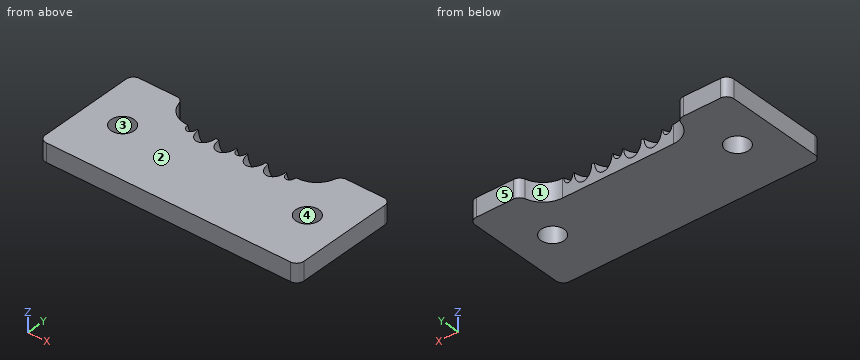
```python
from build123d import *

# Parameters (mm, degrees)
SKETCH1_R               = 3.96875
BOSS_EXTRUDE1_DEPTH     = 6.35
SKETCH2_R               = 3
SKETCH2_R_2             = 1.5875
CUT_EXTRUDE1_DEPTH      = 22.326340521
CUT_EXTRUDE1_DEPTH_BACK = 11.104555903


with BuildPart() as part:
    # Sketch1 → Boss-Extrude1 (new body)
    with BuildSketch(Plane.XY):
        with BuildLine():
            ThreePointArc((17.691011583, 36.198659004), (20.503728332, 31.849390129), (25.4, 30.16))
            Line((25.4, 30.16), (63.5, 30.16))
            ThreePointArc((63.5, 30.16), (68.396271668, 31.849390129), (71.208988417, 36.198659004))
            ThreePointArc((71.208988417, 36.198659004), (72.094604522, 37.568076156), (73.636251773, 38.1))
            Line((73.636251773, 38.1), (86.4, 38.1))
            ThreePointArc((86.4, 38.1), (88.167766953, 37.367766953), (88.9, 35.6))
            Line((88.9, 35.6), (88.9, 2.5))
            ThreePointArc((88.9, 2.5), (88.167766953, 0.732233047), (86.4, 0))
            Line((86.4, 0), (2.5, 0))
            ThreePointArc((2.5, 0), (0.732233047, 0.732233047), (0, 2.5))
            Line((0, 2.5), (0, 35.6))
            ThreePointArc((0, 35.6), (0.732233047, 37.367766953), (2.5, 38.1))
            Line((2.5, 38.1), (15.263748227, 38.1))
            ThreePointArc((15.263748227, 38.1), (16.805395478, 37.568076156), (17.691011583, 36.198659004))
        make_face()
        with Locations((12.7, 19.05)):
            Circle(SKETCH1_R, mode=Mode.SUBTRACT)
        with Locations((76.2, 19.05)):
            Circle(SKETCH1_R, mode=Mode.SUBTRACT)
    extrude(amount=BOSS_EXTRUDE1_DEPTH)

    # Sketch2 → Cut-Extrude1 (cut, two sides)
    with BuildSketch(Plane(origin=(0, 11.905, -11.905), x_dir=(1, 0, 0), z_dir=(0, -0.707106781, 0.707106781))) as cut_extrude1_sk:
        with Locations((49.45, 25.816468581)):
            Circle(SKETCH2_R)
        with Locations((39.45, 25.816468581)):
            Circle(SKETCH2_R)
        with Locations((32.45, 25.816468581)):
            Circle(SKETCH2_R)
        with Locations((56.45, 25.816468581)):
            Circle(SKETCH2_R)
        with Locations((61.45, 25.816468581)):
            Circle(SKETCH2_R_2)
        with Locations((27.45, 25.816468581)):
            Circle(SKETCH2_R_2)
        with Locations((44.45, 25.816468581)):
            Circle(SKETCH2_R_2)
    extrude(amount=CUT_EXTRUDE1_DEPTH, mode=Mode.SUBTRACT)
    extrude(cut_extrude1_sk.sketch, amount=-CUT_EXTRUDE1_DEPTH_BACK, mode=Mode.SUBTRACT)


solid = part.part
```
For this review, take the finished solid that the model builds, in its own axes (mm). Face numbers are marked on the shaded views. A direction names the side the tool comes from. Give positions to 0.01 mm unless a question says otherwise; leave off trailing zeros. Order: outer loops, then holes, each group sorted by start corner. A loop starts at its lowest first (then second) coordinate and runs counter-clockwise, first axis right, second up.
1) Take a section at C-C (z = 1). Give the boundary of the cut face in (x, y).
2) Take a section at D-D (y = 33). Give the boundary of the cut face in (x, z), then the cut area to 3 significant figures.
3) The part is to be moulded in two halves that separate along X. For the marked faces 3, 4 and 5, say which applies: released by +X, released by -X, zero draft, split by the parting line, or undercut.
4) Insertion check: pin 1 (6.5 mm diameter, centred on x = 12.7, y = 19.05, fed in from -Z); pin 2 (3 mm diameter, centred on x = 50, z = 2.5, fed in from +Y). Each pin has a flat end and moves straight along its axis. Give the tip position at first contact, or say it passes through.
5) For the marked faces 1 and 2, list the 3-axis set-ups (+Z, -Z, +X, -X, +Y, -Y) from which the entire face can be reached by the end or side of a thin tool; tool diameter is ignored.
6) Wall thickness on line 1 (Y direction, x = 12.7, z = 1.5); line 2 (Y direction, x = 38, z = 1.5); line 3 (X direction, y = 17, z = 5.75): over which ranges is each line inside the solid? List them lowest first.
7) Take a section at A-A (x = 12.7). Give the boundary of the cut face in (y, z).
8) Take a section at B-B (y = 19.05). Give the boundary of the cut face in (x, z), then the cut area to 3 significant figures.
Derived:
1. outline: (0, 2.5) arc R2.5 ccw to (2.5, 0) - (86.4, 0) arc R2.5 ccw to (88.9, 2.5) - (88.9, 35.6) arc R2.5 ccw to (86.4, 38.1) - (73.64, 38.1) arc R2.5 ccw to (71.21, 36.2) arc R7.94 cw to (63.5, 30.16) - (25.4, 30.16) arc R7.94 cw to (17.69, 36.2) arc R2.5 ccw to (15.26, 38.1) - (2.5, 38.1) arc R2.5 ccw to (0, 35.6) - close; hole circle Ø7.94 at (12.7, 19.05); hole circle Ø7.94 at (76.2, 19.05)
2. outline: (0, 0) - (19.31, 0) - (19.31, 6.35) - (0, 6.35) - close; (69.59, 0) - (88.9, 0) - (88.9, 6.35) - (69.59, 6.35) - close
2. area: 245 mm2
3. face 3: undercut
3. face 4: undercut
3. face 5: zero draft
4. pin 1: passes through
4. pin 2: stops at y = 30.16
5. face 1: +Z, -Z, +Y
5. face 2: +Z, +X, -X, +Y, -Y
6. line 1: y = 0 to 15.08, 23.02 to 38.1
6. line 2: y = 0 to 30.16
6. line 3: x = 0 to 9.3, 16.1 to 72.8, 79.6 to 88.9
7. outline: (0, 0) - (15.08, 0) - (15.08, 6.35) - (0, 6.35) - close; (23.02, 0) - (38.1, 0) - (38.1, 6.35) - (23.02, 6.35) - close
8. outline: (0, 0) - (8.73, 0) - (8.73, 6.35) - (0, 6.35) - close; (16.67, 0) - (72.23, 0) - (72.23, 6.35) - (16.67, 6.35) - close; (80.17, 0) - (88.9, 0) - (88.9, 6.35) - (80.17, 6.35) - close
8. area: 464 mm2
